Source: CAD feature listing. Evaluate the final solid. Frame: model axes, mm. Face numbers are marked on the shaded views. Give positions to 0.01 mm unless a question says otherwise; leave off trailing zeros. Order: outer loops, then holes, each group sorted by start corner. A loop starts at its lowest first (then second) coordinate and runs counter-clockwise, first axis right, second up. Notation, with made-up numbers: (24.5, -32.5) - (50.5, -32.5) arc R23 cw to (50.5, -21.5) - close; hole circle Ø10 at (81, -20.5). An arc over 180 degrees is marked (long way). Use CSV: the item, a comma, the result in double quotes.
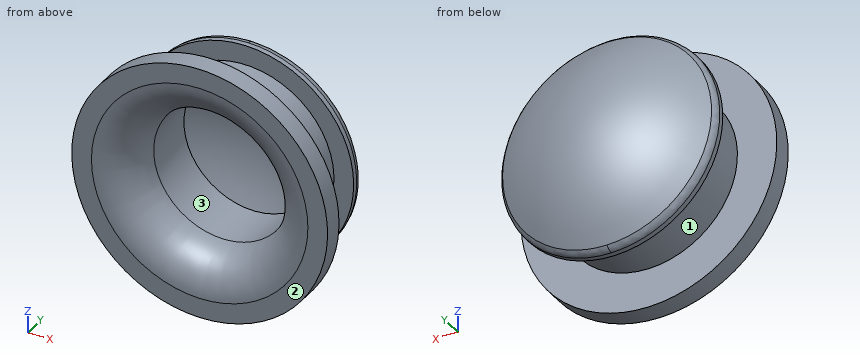
```python
from build123d import *

# Parameters (mm, degrees)
D_ME1_FACE_RADIUS = 5.5
D_ME1_HEIGHT      = 2
CONG_1_R          = 0.5
CONG_2_R          = 2


# Read off the part's stored shape, not the designer's step: Coque1
with BuildPart() as part:
    # Esquisse1 → Révolution1 (revolve)
    with BuildSketch(Plane.XY, mode=Mode.PRIVATE) as r_volution1_sk:
        Polygon((0, 0), (0, 4.5), (5.5, 4.5), (5.5, 4), (4.5, 4), (4.5, 1), (6.5, 1), (6.5, 0), align=None)
    revolve(r_volution1_sk.sketch.rotate(Axis((0, 0, 0), (0, 1, 0)), 90), axis=Axis((0, 0, 0), (0, 1, 0)))

    # Dôme1: a dome of height H over a round flat face of radius A is a cap of a sphere of radius (A * A + H * H) / (2 * H)
    d_me1_r = (D_ME1_FACE_RADIUS * D_ME1_FACE_RADIUS + D_ME1_HEIGHT * D_ME1_HEIGHT) / (2 * D_ME1_HEIGHT)
    d_me1_base = Plane((0, 4.5, 0), z_dir=(0, 1, 0))
    with Locations(d_me1_base.offset(D_ME1_HEIGHT - d_me1_r)):
        d_me1_ball = Sphere(d_me1_r, mode=Mode.PRIVATE)
    add(split(d_me1_ball, bisect_by=d_me1_base, keep=Keep.TOP, mode=Mode.PRIVATE))

    # Congé1
    cong_1_edges = [part.edges().sort_by_distance(p)[0] for p in [
        (5.5, 4.5, 0),
    ]]
    fillet(cong_1_edges, radius=CONG_1_R)

    # Coque1 outline → Coque1 (revolve, cut)
    with BuildSketch(Plane.XY):
        with BuildLine():
            Line((3.5, 0), (3.500000007, 4.641335186))
            ThreePointArc((3.500000007, 4.641335186), (1.801895205, 5.282197402), (0, 5.5))
            Line((0, 5.5), (0, 0))
            Line((0, 0), (3.5, 0))
        make_face()
    revolve(axis=Axis((0, 0, 0), (0, 1, 0)), mode=Mode.SUBTRACT)

    # Congé2
    cong_2_edges = [part.edges().sort_by_distance(p)[0] for p in [
        (-3.5, 0, 0),
    ]]
    fillet(cong_2_edges, radius=CONG_2_R)


solid = part.part
```
Item 1: Section C-C on y = 6.25. Return the cut outline in (x, z).
Filled in:
outline,"circle Ø4.11 at (0, 0)"
Item 2: Material intervals for line 1 (X direction, y = 3.8, z = 0); line 2 (Z direction, x = 3.25, y = 0.5); line 3 (X direction, y = 4.25, z = -1.75), sorted ascending. Write a range as from..to.
Filled in:
line 1,"x = -4.5..-3.5, 3.5..4.5"
line 2,"z = -5.63..-2.62, 2.62..5.63"
line 3,"x = -5.21..-3.03, 3.03..5.21"
Item 3: Section A-A on y = 3.75. Return the cut outline in (x, z).
Filled in:
outline,"circle Ø9 at (0, 0); hole circle Ø7 at (0, 0)"
Item 4: Mould query, pull axis X, two halves, no side actions, for the marked faces 1, 2 and 3. Classes: released by +X, released by -X, zero draft, split by the parting line, or undercut.
Filled in:
face 1,"split by the parting line"
face 2,"zero draft"
face 3,"undercut"
Item 5: Section B-B on x = 5.75. Return the cut outline in (y, z), then the cut area to 3 significant figures.
Filled in:
outline,"(0, -3.03) - (1, -3.03) - (1, 3.03) - (0, 3.03) - close"
area,"6.06 mm2"
Item 6: First-contact query: pin 1 (1.5 mm diameter, centred on x = 4.5, y = 2, fed in from -Z); pin 2 (6 mm diameter, centred on x = 1, z = -5, fed in from -Y); pin 3 (5.5 mm diameter, centred on x = 2, z = 0, fed in from -Y); pin 4 (1 mm diameter, centred on x = -2, y = 3, fed in from +Z). Flat tips, straight axial feed; report the tip coordinate or a pass-through.
Filled in:
pin 1,"stops at z = -2.49"
pin 2,"stops at y = 0"
pin 3,"stops at y = 0.15"
pin 4,"stops at z = 4.24"
